from build123d import *

# Parameters (mm, degrees)
SKETCH_1_W          = 82
SKETCH_1_H          = 71
SKETCH_1_R          = 3
SKETCH_1_W_2        = 66
SKETCH_1_H_2        = 55
EXTRUDE_1_DEPTH     = 20
SKETCH_1_3_R        = 3
CUT_EXTRUDE_1_DEPTH = 20


with BuildPart() as part:
    # 草图1 → 凸台-拉伸1 (new body)
    with BuildSketch(Plane.XY):
        Rectangle(SKETCH_1_W, SKETCH_1_H)
        with Locations((-36, 30.5)):
            Circle(SKETCH_1_R, mode=Mode.SUBTRACT)
        with Locations((-36, -30.5)):
            Circle(SKETCH_1_R, mode=Mode.SUBTRACT)
        Rectangle(SKETCH_1_W_2, SKETCH_1_H_2, mode=Mode.SUBTRACT)
    extrude(amount=EXTRUDE_1_DEPTH)

    # 草图1<3> → 切除-拉伸1 (cut)
    with BuildSketch(Plane.XY):
        with Locations((36, -30.5)):
            Circle(SKETCH_1_3_R)
        with Locations((36, 30.5)):
            Circle(SKETCH_1_3_R)
    extrude(amount=CUT_EXTRUDE_1_DEPTH, mode=Mode.SUBTRACT)


solid = part.part
Design review of the part built by this model. Coordinates are the model's own, in mm. A direction names the side the tool comes from. Round coordinates to 2 decimals unless told otherwise and drop trailing zeros. Loops run counter-clockwise (first coordinate to the right, second up) from the corner with the lowest first, then second, coordinate; pieces in that order, holes last. Notation, with made-up numbers: (57.25, -38.75) - (62.25, -38.75) arc R10 ccw to (62.25, -29.75) - close; hole circle Ø6 at (62, 50). An arc over 180 degrees is marked (long way). One line per item, written item: value. Start each with the question number.
1) Consider section C-C on y = -30.5. Give the boundary of the cut face in (x, z).
2) To check wall thickness, follow L1, parallel to Y at x = -36, z = 8.5; L2, parallel to Y at x = -26, z = 8.75; L3, parallel to X at y = 9, z = 16. State the ranges of each line that lie inside material, in increasing order. Write a range as from..to.
3) Consider section D-D on x = 36. Give the boundary of the cut face in (y, z), then the cut area to 3 significant figures.
4) For faces 5 (the flat face through (-33, 0, 10)), 6 (the flat face through (-1, 35.5, 10)), list the 3-axis set-ups (+Z, -Z, +X, -X, +Y, -Y) from which the entire face can be reached by the end or side of a thin tool; tool diameter is ignored.
5) Consider section B-B on z = 11.5. Give the boundary of the cut face in (x, y), then the cut area to 3 significant figures.
6) Insertion check: pin 1 Ø3.5 at (x, y) = (-36, 30.5) entering from -Z. The pin has a flat end and moves straight along its axis. Give the tip position at first contact, or say it passes through.
7) Consider section A-A on y = 15. Give the boundary of the cut face in (x, z).
8) Draft analysis for pull direction Y (two halves, no side actions). For faces 1 (the flat face through (-41, 0, 10)), 2 (the cylindrical face through (-39, 30.6, 9.9)), 3 (the flat face through (33, 0, 10)), 4 (the flat face through (-1, -35.5, 10)), state which applies: +Y half, -Y half, draft (parallel to the pull), parting line (faces both ways), or undercut.
Reported:
1. outline: (-41, 0) - (-39, 0) - (-39, 20) - (-41, 20) - close; (-33, 0) - (33, 0) - (33, 20) - (-33, 20) - close; (39, 0) - (41, 0) - (41, 20) - (39, 20) - close
2. L1: y = -35.5..-33.5, -27.5..27.5, 33.5..35.5
2. L2: y = -35.5..-27.5, 27.5..35.5
2. L3: x = -41..-33, 33..41
3. outline: (-35.5, 0) - (-33.5, 0) - (-33.5, 20) - (-35.5, 20) - close; (-27.5, 0) - (27.5, 0) - (27.5, 20) - (-27.5, 20) - close; (33.5, 0) - (35.5, 0) - (35.5, 20) - (33.5, 20) - close
3. area: 1,180 mm^2
4. face 5: +Z, -Z
4. face 6: +Z, -Z, +X, -X, +Y
5. outline: (-41, -35.5) - (41, -35.5) - (41, 35.5) - (-41, 35.5) - close; hole circle Ø6 at (-36, -30.5); hole circle Ø6 at (-36, 30.5); hole (-33, -27.5) - (33, -27.5) - (33, 27.5) - (-33, 27.5) - close; hole circle Ø6 at (36, -30.5); hole circle Ø6 at (36, 30.5)
5. area: 2,080 mm^2
6. pin 1: passes through
7. outline: (-41, 0) - (-33, 0) - (-33, 20) - (-41, 20) - close; (33, 0) - (41, 0) - (41, 20) - (33, 20) - close
8. face 1: draft
8. face 2: undercut
8. face 3: undercut
8. face 4: -Y half
